```python
from build123d import *

# Parameters (mm, degrees)
BOSS_EXTRUDE1_DEPTH = 7.9375
SKETCH2_R           = 5.207
CUT_EXTRUDE1_DEPTH  = 3.96875
SKETCH4_W           = 5.08
SKETCH4_H           = 15.875
BOSS_EXTRUDE2_DEPTH = 20.32


with BuildPart() as part:
    # Sketch1 → Boss-Extrude1 (new, symmetric)
    with BuildSketch(Plane(origin=(0, 0, 0), x_dir=(1, 0, 0), z_dir=(0, 1, 0))):
        Polygon((0, 0), (3.96875, 0), (120.93575, 0), (120.93575, 3.96875), (3.96875, 3.96875), (3.96875, 75.34275), (0, 75.34275), align=None)
    extrude(amount=BOSS_EXTRUDE1_DEPTH, both=True)

    # Sketch2 → Cut-Extrude1 (cut)
    with BuildSketch(Plane.XY):
        with Locations((73.50125, 0)):
            Circle(SKETCH2_R)
    extrude(amount=-CUT_EXTRUDE1_DEPTH, mode=Mode.SUBTRACT)

    # Sketch4 → Boss-Extrude2 (add)
    with BuildSketch(Plane.XY):
        with Locations((53.68925, 0)):
            Rectangle(SKETCH4_W, SKETCH4_H)
        with Locations((81.88325, 0)):
            Rectangle(SKETCH4_W, SKETCH4_H)
    extrude(amount=BOSS_EXTRUDE2_DEPTH)


solid = part.part
```
Part model, mm, in its own coordinate system. A direction names the side the tool comes from. Give positions to 0.01 mm unless a question says otherwise; leave off trailing zeros. Order: outer loops, then holes, each group sorted by start corner. A loop starts at its lowest first (then second) coordinate and runs counter-clockwise, first axis right, second up. Notation, with made-up numbers: M 77.25,-32 L 131.25,-32 A21 cw 131.25,-14 Z; hole C 35.5,66 d10. An arc over 180 degrees is marked long. Use a Markdown table: item, result. Add a question column.
(1) Drop flat-ended pins along their axis: P1, Ø3, axis at y = 6, z = -65, coming from the +X side; P2, Ø5, axis at y = 0.5, z = 13, coming from the +X side; P3, Ø8, axis at y = 2.5, z = 6, coming from the -X side. Give the stop position or say it passes through.
(2) Saw through at A-A, the plane y = 3.75. Give the cut face in (x, z).
(3) Saw through at B-B, the plane z = -34.5. Give the cut face in (x, y).
(4) Mould opens along X. For faces 4 (the face through (82, 0, 20.32)), 5 (the face through (84.423, 0, 10)), 6 (the face through (68.3, 0.2, -2)) say: +X half, -X half, draft (parallel to the pull), parting line (faces both ways), or undercut.
(5) Saw through at C-C, the plane x = 10.5. Give the cut face in (y, z), and give its area (3 significant figures).
(6) Probe line 1 along X through (y, z) = (-2.5, 3.5); line 2 along X through (y, z) = (1, -48); line 3 along Z through (x, y) = (40, -1.5). List the from-to ranges inside material, lowest first. Write a range as [from, to].
(7) 3-axis set-ups, long thin cutter, end or side, ignore diameter. For faces 1 (the face through (51.149, 0, 10)), 2 (the face through (65, 0, 0)), 3 (the face through (102, 0, 0)): which of +Z, -Z, +X, -X, +Y, -Y reach the whole face in a straight line?
Answer key:
| question | item | result |
|---|---|---|
| 1 | P1 | x = 3.97 |
| 1 | P2 | x = 84.42 |
| 1 | P3 | x = 51.15 |
| 2 | outline | M 0,-75.34 L 3.97,-75.34 L 3.97,-3.97 L 69.89,-3.97 L 69.89,0 L 56.23,0 L 56.23,20.32 L 51.15,20.32 L 51.15,0 L 0,0 Z; M 77.11,-3.97 L 120.94,-3.97 L 120.94,0 L 84.42,0 L 84.42,20.32 L 79.34,20.32 L 79.34,0 L 77.11,0 Z |
| 3 | outline | M 0,-7.94 L 3.97,-7.94 L 3.97,7.94 L 0,7.94 Z |
| 4 | face 4 | draft |
| 4 | face 5 | +X half |
| 4 | face 6 | undercut |
| 5 | outline | M -7.94,-3.97 L 7.94,-3.97 L 7.94,0 L -7.94,0 Z |
| 5 | area | 63.0 mm^2 |
| 6 | line 1 | [51.15, 56.23], [79.34, 84.42] |
| 6 | line 2 | [0, 3.97] |
| 6 | line 3 | [-3.97, 0] |
| 7 | face 1 | +Z, -X, +Y, -Y |
| 7 | face 2 | +Z, +Y, -Y |
| 7 | face 3 | +Z, +X, +Y, -Y |
